```python
from build123d import *

# Parameters (mm, degrees)
SKETCH1_W           = 583
SKETCH1_H           = 408
BOSS_EXTRUDE1_DEPTH = 11
SKETCH2_W           = 583
SKETCH2_H           = 408
SKETCH2_W_2         = 577
SKETCH2_H_2         = 402
BOSS_EXTRUDE2_DEPTH = 1
SKETCH3_W           = 583
SKETCH3_H           = 408
SKETCH3_W_2         = 577
SKETCH3_H_2         = 402
BOSS_EXTRUDE3_DEPTH = 1
FILLET2_R           = 40


with BuildPart() as part:
    # Sketch1 → Boss-Extrude1 (new body)
    with BuildSketch(Plane(origin=(0, 0, 0), x_dir=(1, 0, 0), z_dir=(0, 1, 0))):
        Rectangle(SKETCH1_W, SKETCH1_H)
    extrude(amount=BOSS_EXTRUDE1_DEPTH)

    # Sketch2 → Boss-Extrude2 (add)
    with BuildSketch(Plane(origin=(0, 11, 0), x_dir=(1, 0, 0), z_dir=(0, 1, 0))):
        Rectangle(SKETCH2_W, SKETCH2_H)
        Rectangle(SKETCH2_W_2, SKETCH2_H_2, mode=Mode.SUBTRACT)
    extrude(amount=BOSS_EXTRUDE2_DEPTH)

    # Sketch3 → Boss-Extrude3 (add)
    with BuildSketch(Plane.XZ):
        Rectangle(SKETCH3_W, SKETCH3_H)
        Rectangle(SKETCH3_W_2, SKETCH3_H_2, mode=Mode.SUBTRACT)
    extrude(amount=BOSS_EXTRUDE3_DEPTH)

    # Fillet2
    fillet2_edges = [part.edges().sort_by_distance(p)[0] for p in [
        (-288.5, 11.5, 201),
        (288.5, 11.5, 201),
        (288.5, 11.5, -201),
        (-288.5, 11.5, -201),
        (-288.5, -0.5, -201),
        (288.5, -0.5, -201),
        (288.5, -0.5, 201),
        (-288.5, -0.5, 201),
        (291.5, 5.5, 204),
        (-291.5, 5.5, 204),
        (-291.5, 5.5, -204),
        (291.5, 5.5, -204),
    ]]
    fillet(fillet2_edges, radius=FILLET2_R)


solid = part.part
```
For this review, take the finished solid that the model builds, in its own axes (mm). A direction names the side the tool comes from. Round coordinates to 2 decimals unless told otherwise and drop trailing zeros. Write each loop counter-clockwise with the first axis right and the second up, starting at its lowest first coordinate (ties: lowest second). Pieces come first, ordered by that corner, then holes. Notation, with made-up numbers: (86, 41) - (142, 41) arc R15 ccw to (142, 67) - close; hole circle Ø10 at (5, 77). An arc over 180 degrees is marked (long way). Use CSV: the item, a comma, the result in double quotes.
1) Clearance check with a flat-ended pin moving along its axis: pin 1 Ø5 at (x, z) = (-86.5, -15.5) entering from +Y. State where the tip first meets the part, or that it passes through.
Conclusion:
pin 1,"stops at y = 11"
2) For faces 1 (the cylindrical face through (-277.094, 11.507, -188.972)), 2 (the flat face through (-4, 0, -3)), 3 (the cylindrical face through (279.472, 5.409, -192.594)), list the 3-axis set-ups (+Z, -Z, +X, -X, +Y, -Y) from which the entire face can be reached by the end or side of a thin tool; tool diameter is ignored.
Conclusion:
face 1,"+Y"
face 2,"-Y"
face 3,"-Z, +X, +Y, -Y"
3) Wall thickness on line 1 along Y through (x, z) = (-160, -65.5); line 2 along X through (y, z) = (-0.5, 109); line 3 along Z through (x, y) = (268, 2.5): over which ranges is each line inside the solid? List them lowest first. Write a range as from..to.
Conclusion:
line 1,"y = 0..11"
line 2,"x = -291.5..-288.5, 288.5..291.5"
line 3,"z = -200.44..200.44"
4) The part is to be moulded in two halves that separate along Z. For faces 4 (the flat face through (-4, 6, -204)), 5 (the cylindrical face through (276.472, -0.507, 189.594)), 6 (the flat face through (-291.5, 6, -2)), 7 (the cylindrical face through (277.094, -0.507, -188.972)), say which applies: pulls with the +Z half, pulls with the -Z half, needs draft (parallel to the pull), parting line crosses it, or undercut.
Conclusion:
face 4,"pulls with the -Z half"
face 5,"undercut"
face 6,"needs draft"
face 7,"undercut"
5) Add section A-A on z = 37. Write out the cut boundary in (x, y).
Conclusion:
outline,"(-291.5, -1) - (-288.5, -1) - (-288.5, 0) - (288.5, 0) - (288.5, -1) - (291.5, -1) - (291.5, 12) - (288.5, 12) - (288.5, 11) - (-288.5, 11) - (-288.5, 12) - (-291.5, 12) - close"
6) Add section B-B on x = -80.5. Write out the cut boundary in (y, z), and give its area (3 significant figures).
Conclusion:
outline,"(-1, -204) - (12, -204) - (12, -201) - (11, -201) - (11, 201) - (12, 201) - (12, 204) - (-1, 204) - (-1, 201) - (0, 201) - (0, -201) - (-1, -201) - close"
area,"4,500 mm^2"
